Read the model definition and answer for the solid it produces. Units are mm, in the model's axes. Face numbers are marked on the shaded views. A direction names the side the tool comes from. Round coordinates to 2 decimals unless told otherwise and drop trailing zeros. Write each loop counter-clockwise with the first axis right and the second up, starting at its lowest first coordinate (ties: lowest second). Pieces come first, ordered by that corner, then holes. Notation, with made-up numbers: M 49,-19 L 81,-19 A17 ccw 81,1 Z; hole C 8,26 d8. An arc over 180 degrees is marked long. Use one line per item in the form item = value. Start each with the question number.
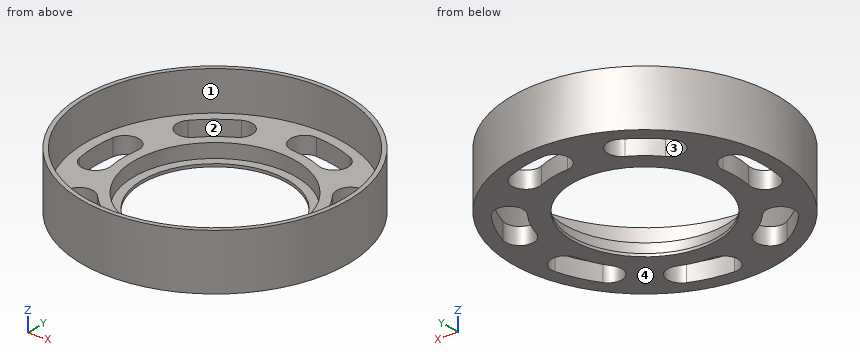
```python
from build123d import *

# Parameters (mm, degrees)
SKETCH1_R           = 47.5
SKETCH1_R_2         = 46
BOSS_EXTRUDE1_DEPTH = 20
SKETCH1_5_R         = 46
SKETCH1_5_R_2       = 29
BOSS_EXTRUDE2_DEPTH = 6
SKETCH1_7_R         = 29
SKETCH1_7_R_2       = 26
BOSS_EXTRUDE4_DEPTH = 1


with BuildPart() as part:
    # Sketch1 → Boss-Extrude1 (new body)
    with BuildSketch(Plane.XY):
        Circle(SKETCH1_R)
        Circle(SKETCH1_R_2, mode=Mode.SUBTRACT)
    extrude(amount=BOSS_EXTRUDE1_DEPTH)

    # Sketch1<5> → Boss-Extrude2 (add)
    with BuildSketch(Plane.XY):
        Circle(SKETCH1_5_R)
        with BuildLine():
            ThreePointArc((-31.865701126, -28.121648098), (-31.425224299, -21.064312895), (-24.367889096, -21.504789722))
            ThreePointArc((-24.367889096, -21.504789722), (-20.26341856, -25.40952318), (-15.543254305, -28.542201135))
            ThreePointArc((-15.543254305, -28.542201135), (-13.543416331, -35.324578894), (-20.325794091, -37.324416868))
            ThreePointArc((-20.325794091, -37.324416868), (-26.498316579, -33.227838005), (-31.865701126, -28.121648098))
        make_face(mode=Mode.SUBTRACT)
        with BuildLine():
            ThreePointArc((2.118450141, -42.447169152), (-3.124563894, -37.702613974), (1.619991284, -32.45959994))
            ThreePointArc((1.619991284, -32.45959994), (7.231930354, -31.685157146), (12.624130879, -29.947976886))
            ThreePointArc((12.624130879, -29.947976886), (19.17368592, -32.613183964), (16.508478842, -39.162739004))
            ThreePointArc((16.508478842, -39.162739004), (9.457139693, -41.434436268), (2.118450141, -42.447169152))
        make_face(mode=Mode.SUBTRACT)
        with BuildLine():
            ThreePointArc((34.507365243, -24.80910607), (27.528956853, -25.950077737), (26.387985186, -18.971669348))
            ThreePointArc((26.387985186, -18.971669348), (29.281488207, -14.101221521), (31.285288026, -8.802315215))
            ThreePointArc((31.285288026, -8.802315215), (37.452611601, -5.343396321), (40.911530495, -11.510719896))
            ThreePointArc((40.911530495, -11.510719896), (38.291176886, -18.440058912), (34.507365243, -24.80910607))
        make_face(mode=Mode.SUBTRACT)
        with BuildLine():
            ThreePointArc((-41.854329503, -7.380047551), (-42.5, 0), (-41.854329503, 7.380047551))
            ThreePointArc((-41.854329503, 7.380047551), (-36.06204985, 11.435845428), (-32.006251973, 5.643565774))
            ThreePointArc((-32.006251973, 5.643565774), (-32.5, 0), (-32.006251973, -5.643565774))
            ThreePointArc((-32.006251973, -5.643565774), (-36.06204985, -11.435845428), (-41.854329503, -7.380047551))
        make_face(mode=Mode.SUBTRACT)
        with BuildLine():
            ThreePointArc((-20.325794091, 37.324416868), (-13.543416331, 35.324578894), (-15.543254305, 28.542201135))
            ThreePointArc((-15.543254305, 28.542201135), (-20.26341856, 25.40952318), (-24.367889096, 21.504789722))
            ThreePointArc((-24.367889096, 21.504789722), (-31.425224299, 21.064312895), (-31.865701126, 28.121648098))
            ThreePointArc((-31.865701126, 28.121648098), (-26.498316579, 33.227838005), (-20.325794091, 37.324416868))
        make_face(mode=Mode.SUBTRACT)
        Circle(SKETCH1_5_R_2, mode=Mode.SUBTRACT)
        with BuildLine():
            ThreePointArc((40.911530495, 11.510719896), (37.452611601, 5.343396321), (31.285288026, 8.802315215))
            ThreePointArc((31.285288026, 8.802315215), (29.281488207, 14.101221521), (26.387985186, 18.971669348))
            ThreePointArc((26.387985186, 18.971669348), (27.528956853, 25.950077737), (34.507365243, 24.80910607))
            ThreePointArc((34.507365243, 24.80910607), (38.291176886, 18.440058912), (40.911530495, 11.510719896))
        make_face(mode=Mode.SUBTRACT)
        with BuildLine():
            ThreePointArc((16.508478842, 39.162739004), (19.17368592, 32.613183964), (12.624130879, 29.947976886))
            ThreePointArc((12.624130879, 29.947976886), (7.231930354, 31.685157146), (1.619991284, 32.45959994))
            ThreePointArc((1.619991284, 32.45959994), (-3.124563894, 37.702613974), (2.118450141, 42.447169152))
            ThreePointArc((2.118450141, 42.447169152), (9.457139693, 41.434436268), (16.508478842, 39.162739004))
        make_face(mode=Mode.SUBTRACT)
    extrude(amount=BOSS_EXTRUDE2_DEPTH)

    # Sketch1<7> → Boss-Extrude4 (add)
    with BuildSketch(Plane.XY):
        Circle(SKETCH1_7_R)
        Circle(SKETCH1_7_R_2, mode=Mode.SUBTRACT)
    extrude(amount=BOSS_EXTRUDE4_DEPTH)


solid = part.part
```
Q1. Straight lines are drawn through the part: line 1 (Y direction, x = 0, z = 2.55); line 2 (Z direction, x = 43.5, y = 5.5); line 3 (Y direction, x = -24, z = 2.5). For each, find the intervals that lie inside material, in ascending order. Write a range as [from, to].
Q2. Find section C-C on x = 23. Write down the section's boundary in (y, z), and give its area (3 significant figures).
Q3. Find section D-D on z = 14.5. Write down the section's boundary in (x, y), and give its area (3 significant figures).
Q4. Find section A-A on y = 0. Write down the section's boundary in (x, z).
Q5. Each of these flat-tipped pins is pushed along its axis until it touches: pin 1 Ø8 at (x, y) = (-26, 8) entering from +Z; pin 2 Ø10 at (x, z) = (-30.5, 11) entering from -Y; pin 3 Ø10 at (x, z) = (-10, 4.5) entering from -Y. Where does it stop, or does it pass through?
Q6. A tool of negligible diameter and unlimited length cuts with its end or side. For the marked faces 1 and 2, from which of +Z, -Z, +X, -X, +Y, -Y can it reach the whole face along a straight path? Write none if from no direction.
Q7. For a pull along Y with two mould halves and no side action, classify the marked faces 3 and 4 as +Y half, -Y half, draft (parallel to the pull), parting line (faces both ways), or undercut.
Q8. Find section B-B on x = -17. Write down the section's boundary in (y, z).
Response:
q1.line_1 = [-47.5, -42.09], [-32.82, -29], [29, 32.82], [42.09, 47.5]
q1.line_2 = [0, 6]
q1.line_3 = [-40.99, -35.07], [-21.91, -16.28], [16.28, 21.91], [35.07, 40.99]
q2.outline = M -41.56,0 L -12.12,0 L -12.12,1 L -17.66,1 L -17.66,6 L -39.84,6 L -39.84,20 L -41.56,20 Z; M 12.12,0 L 41.56,0 L 41.56,20 L 39.84,20 L 39.84,6 L 17.66,6 L 17.66,1 L 12.12,1 Z
q2.area = 346 mm²
q3.outline = C 0,0 d95; hole C 0,0 d92
q3.area = 441 mm²
q4.outline = M -47.5,0 L -42.5,0 L -42.5,6 L -46,6 L -46,20 L -47.5,20 Z; M -32.5,0 L -26,0 L -26,1 L -29,1 L -29,6 L -32.5,6 Z; M 26,0 L 47.5,0 L 47.5,20 L 46,20 L 46,6 L 29,6 L 29,1 L 26,1 Z
q5.pin_1 = 6
q5.pin_2 = -40.07
q5.pin_3 = -47.24
q6.face_1 = +Z
q6.face_2 = +Z, -Z
q7.face_3 = undercut
q7.face_4 = draft
q8.outline = M -44.35,0 L -37.85,0 L -37.85,6 L -42.74,6 L -42.74,20 L -44.35,20 Z; M -27.7,0 L -19.67,0 L -19.67,1 L -23.49,1 L -23.49,6 L -27.7,6 Z; M 19.67,0 L 27.7,0 L 27.7,6 L 23.49,6 L 23.49,1 L 19.67,1 Z; M 37.85,0 L 44.35,0 L 44.35,20 L 42.74,20 L 42.74,6 L 37.85,6 Z
